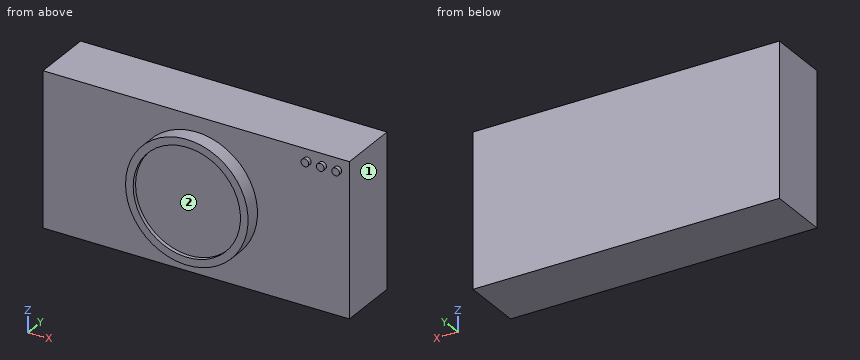
```python
from build123d import *

# Parameters (mm, degrees)
SKETCH1_W           = 20
SKETCH1_H           = 4
BOSS_EXTRUDE1_DEPTH = 10
SKETCH2_R           = 4
BOSS_EXTRUDE2_DEPTH = 1
SKETCH5_R           = 3.5
CUT_EXTRUDE1_DEPTH  = 0.25
SKETCH6_R           = 0.25
BOSS_EXTRUDE3_DEPTH = 0.25


with BuildPart() as part:
    # Sketch1 → Boss-Extrude1 (new body)
    with BuildSketch(Plane.XY):
        Rectangle(SKETCH1_W, SKETCH1_H)
    extrude(amount=BOSS_EXTRUDE1_DEPTH)

    # Sketch2 → Boss-Extrude2 (add)
    with BuildSketch(Plane(origin=(0, -2, 0), x_dir=(-1, 0, 0), z_dir=(0, -1, 0))):
        with Locations((0, -5)):
            Circle(SKETCH2_R)
    extrude(amount=BOSS_EXTRUDE2_DEPTH)

    # Sketch5 → Cut-Extrude1 (cut)
    with BuildSketch(Plane(origin=(0, -3, 0), x_dir=(-1, 0, 0), z_dir=(0, -1, 0))):
        with Locations((0, -5)):
            Circle(SKETCH5_R)
    extrude(amount=-CUT_EXTRUDE1_DEPTH, mode=Mode.SUBTRACT)

    # Sketch6 → Boss-Extrude3 (add)
    with BuildSketch(Plane(origin=(0, -2, 0), x_dir=(-1, 0, 0), z_dir=(0, -1, 0))):
        with Locations((-7.25, -9.25)):
            Circle(SKETCH6_R)
        with Locations((-8.25, -9.25)):
            Circle(SKETCH6_R)
        with Locations((-9.25, -9.25)):
            Circle(SKETCH6_R)
    extrude(amount=BOSS_EXTRUDE3_DEPTH)


solid = part.part
```
The listing builds one solid part. Answer for the finished solid, in the listing's coordinates (mm). Face numbers are marked on the shaded views. A direction names the side the tool comes from. Round coordinates to 2 decimals unless told otherwise and drop trailing zeros. Write each loop counter-clockwise with the first axis right and the second up, starting at its lowest first coordinate (ties: lowest second). Pieces come first, ordered by that corner, then holes. Notation, with made-up numbers: (86.5, 78) -> (135.5, 78) arc R24 ccw to (135.5, 113) -> close; hole circle Ø5 at (-26.5, -27.75). An arc over 180 degrees is marked (long way). Answer as a JSON object with one key per item and string values. Group by question number.
Q1. Section D-D (z = 9.25) is taken. Write down the section's boundary in (x, y), plus the area to 3 significant figures.
Q2. Section A-A (x = 0) is taken. Write down the section's boundary in (y, z).
Q3. Section B-B (z = 5) is taken. Write down the section's boundary in (x, y).
Q4. Each of these flat-tipped pins is pushed along its axis until it touches: pin 1 Ø3.5 at (x, z) = (0, 6) entering from -Y; pin 2 Ø0.6 at (x, z) = (8.5, 9.5) entering from -Y. Where does it stop, or does it pass through?
Q5. Straight lines are drawn through the part: line 1 along Z through (x, y) = (0, -2.85); line 2 along X through (y, z) = (-2.8, 5); line 3 along Y through (x, z) = (4.25, 1.75). For each, find the intervals that lie inside material, in ascending order.
Q6. Section C-C (x = 9.25) is taken. Write down the section's boundary in (y, z), plus the area to 3 significant figures.
Q7. Which of the six approach directions +Z, -Z, +X, -X, +Y, -Y give full straight-line access (tool end or side, diameter ignored) to the marked faces 1 and 2?
Check values:
{
 "1": {"outline": "(-10, -2) -> (7, -2) -> (7, -2.25) -> (7.5, -2.25) -> (7.5, -2) -> (8, -2) -> (8, -2.25) -> (8.5, -2.25) -> (8.5, -2) -> (9, -2) -> (9, -2.25) -> (9.5, -2.25) -> (9.5, -2) -> (10, -2) -> (10, 2) -> (-10, 2) -> close", "area": "80.4 mm^2"},
 "2": {"outline": "(-3, 1) -> (-2, 1) -> (-2, 0) -> (2, 0) -> (2, 10) -> (-2, 10) -> (-2, 9) -> (-3, 9) -> (-3, 8.5) -> (-2.75, 8.5) -> (-2.75, 1.5) -> (-3, 1.5) -> close"},
 "3": {"outline": "(-10, -2) -> (-4, -2) -> (-4, -3) -> (-3.5, -3) -> (-3.5, -2.75) -> (3.5, -2.75) -> (3.5, -3) -> (4, -3) -> (4, -2) -> (10, -2) -> (10, 2) -> (-10, 2) -> close"},
 "4": {"pin 1": "y = -2.75", "pin 2": "y = -2.25"},
 "5": {"line 1": "1 to 1.5, 8.5 to 9", "line 2": "-4 to -3.5, 3.5 to 4", "line 3": "-2 to 2"},
 "6": {"outline": "(-2.25, 9) -> (-2, 9) -> (-2, 0) -> (2, 0) -> (2, 10) -> (-2, 10) -> (-2, 9.5) -> (-2.25, 9.5) -> close", "area": "40.1 mm^2"},
 "7": {"face 1": "+Z, -Z, +X, +Y, -Y", "face 2": "-Y"}
}
